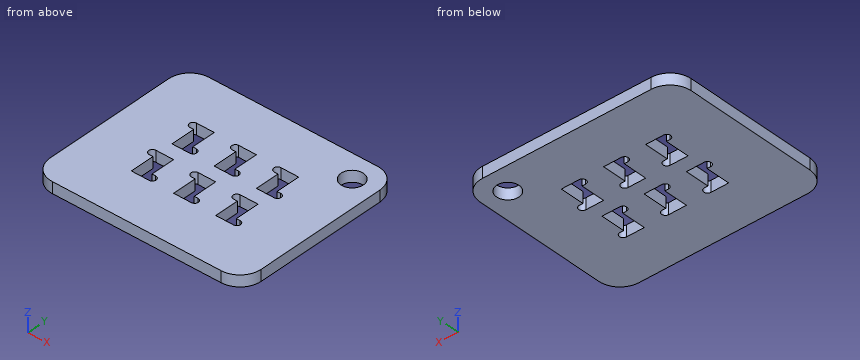
from build123d import *

# Parameters (mm, degrees)
F0_R     = 1.5875
F1_DEPTH = 1.5875


# Not quite as in the source:
# - a length typed as a fraction of an inch, garbled in the dataset ("3 / 203.2 mm" for 3/8 in), is restored


with BuildPart() as f1:
    # F0 (on Top) → F1 (new body)
    with BuildSketch(Plane.XY):
        with BuildLine():
            Line((-6, -12.5), (18, -12.5))
            ThreePointArc((18, -12.5), (20.1213203436, -11.6213203436), (21, -9.5))
            Line((21, -9.5), (21, 9.5))
            ThreePointArc((21, 9.5), (20.1213203436, 11.6213203436), (18, 12.5))
            Line((18, 12.5), (-6, 12.5))
            ThreePointArc((-6, 12.5), (-8.1213203436, 11.6213203436), (-9, 9.5))
            Line((-9, 9.5), (-9, -9.5))
            ThreePointArc((-9, -9.5), (-8.1213203436, -11.6213203436), (-6, -12.5))
        make_face()
        with BuildLine():
            Line((1.525, -5.5), (1, -5.5))
            Line((1, -5.5), (-1, -5.5))
            Line((-1, -5.5), (-1, -2.05))
            Line((-1, -2.05), (-1.525, -2.05))
            ThreePointArc((-1.525, -2.05), (-2.05, -1.525), (-1.525, -1))
            Line((-1.525, -1), (-1, -1))
            Line((-1, -1), (1, -1))
            Line((1, -1), (1, -4.45))
            Line((1, -4.45), (1.525, -4.45))
            ThreePointArc((1.525, -4.45), (2.05, -4.975), (1.525, -5.5))
        make_face(mode=Mode.SUBTRACT)
        with BuildLine():
            Line((7.525, -5.5), (7, -5.5))
            Line((7, -5.5), (5, -5.5))
            Line((5, -5.5), (5, -2.05))
            Line((5, -2.05), (4.475, -2.05))
            ThreePointArc((4.475, -2.05), (3.95, -1.525), (4.475, -1))
            Line((4.475, -1), (5, -1))
            Line((5, -1), (7, -1))
            Line((7, -1), (7, -4.45))
            Line((7, -4.45), (7.525, -4.45))
            ThreePointArc((7.525, -4.45), (8.05, -4.975), (7.525, -5.5))
        make_face(mode=Mode.SUBTRACT)
        with BuildLine():
            Line((13.525, -5.5), (13, -5.5))
            Line((13, -5.5), (11, -5.5))
            Line((11, -5.5), (11, -2.05))
            Line((11, -2.05), (10.475, -2.05))
            ThreePointArc((10.475, -2.05), (9.95, -1.525), (10.475, -1))
            Line((10.475, -1), (11, -1))
            Line((11, -1), (13, -1))
            Line((13, -1), (13, -4.45))
            Line((13, -4.45), (13.525, -4.45))
            ThreePointArc((13.525, -4.45), (14.05, -4.975), (13.525, -5.5))
        make_face(mode=Mode.SUBTRACT)
        with BuildLine():
            Line((-1, 5.5), (1, 5.5))
            Line((1, 5.5), (1, 2.05))
            Line((1, 2.05), (1.525, 2.05))
            ThreePointArc((1.525, 2.05), (2.05, 1.525), (1.525, 1))
            Line((1.525, 1), (1, 1))
            Line((1, 1), (-1, 1))
            Line((-1, 1), (-1, 4.45))
            Line((-1, 4.45), (-1.525, 4.45))
            ThreePointArc((-1.525, 4.45), (-2.05, 4.975), (-1.525, 5.5))
            Line((-1.525, 5.5), (-1, 5.5))
        make_face(mode=Mode.SUBTRACT)
        with BuildLine():
            Line((7.525, 1), (7, 1))
            Line((7, 1), (5, 1))
            Line((5, 1), (5, 4.45))
            Line((5, 4.45), (4.475, 4.45))
            ThreePointArc((4.475, 4.45), (3.95, 4.975), (4.475, 5.5))
            Line((4.475, 5.5), (5, 5.5))
            Line((5, 5.5), (7, 5.5))
            Line((7, 5.5), (7, 2.05))
            Line((7, 2.05), (7.525, 2.05))
            ThreePointArc((7.525, 2.05), (8.05, 1.525), (7.525, 1))
        make_face(mode=Mode.SUBTRACT)
        with BuildLine():
            Line((13.525, 1), (13, 1))
            Line((13, 1), (11, 1))
            Line((11, 1), (11, 4.45))
            Line((11, 4.45), (10.475, 4.45))
            ThreePointArc((10.475, 4.45), (9.95, 4.975), (10.475, 5.5))
            Line((10.475, 5.5), (11, 5.5))
            Line((11, 5.5), (13, 5.5))
            Line((13, 5.5), (13, 2.05))
            Line((13, 2.05), (13.525, 2.05))
            ThreePointArc((13.525, 2.05), (14.05, 1.525), (13.525, 1))
        make_face(mode=Mode.SUBTRACT)
        with Locations((17.5, 9)):
            Circle(F0_R, mode=Mode.SUBTRACT)
    extrude(amount=F1_DEPTH)


solid = f1.part
Read the model definition and answer for the solid it produces. Units are mm, in the model's axes. Give positions to 0.01 mm unless a question says otherwise; leave off trailing zeros. Write each loop counter-clockwise with the first axis right and the second up, starting at its lowest first coordinate (ties: lowest second). Pieces come first, ordered by that corner, then holes. Notation, with made-up numbers: (46, 9.25) - (77, 9.25) arc R22 ccw to (77, 15.25) - close; hole circle Ø1 at (87, -31.5). An arc over 180 degrees is marked (long way). Return JSON: item names as keys, results as strings.
Q1. A cutting plane is placed at C-C, the plane y = 9. Determine the outline of the cut face in (x, z), and give its area (3 significant figures).
Reply:
{"outline": "(-9, 0) - (15.91, 0) - (15.91, 1.59) - (-9, 1.59) - close; (19.09, 0) - (21, 0) - (21, 1.59) - (19.09, 1.59) - close", "area": "42.6 mm²"}
Q2. A cutting plane is placed at A-A, the plane y = 3.25. Determine the outline of the cut face in (x, z).
Reply:
{"outline": "(-9, 0) - (-1, 0) - (-1, 1.59) - (-9, 1.59) - close; (1, 0) - (5, 0) - (5, 1.59) - (1, 1.59) - close; (7, 0) - (11, 0) - (11, 1.59) - (7, 1.59) - close; (13, 0) - (21, 0) - (21, 1.59) - (13, 1.59) - close"}
Q3. A cutting plane is placed at B-B, the plane x = 17.5. Determine the outline of the cut face in (y, z).
Reply:
{"outline": "(-12.5, 0) - (7.41, 0) - (7.41, 1.59) - (-12.5, 1.59) - close; (10.59, 0) - (12.5, 0) - (12.5, 1.59) - (10.59, 1.59) - close"}
Q4. A cutting plane is placed at D-D, the plane z = 0.75. Count the separate pieces of the cut face and the enclosed holes in it, and give its area (3 significant figures).
Reply:
{"separate pieces": "1", "enclosed holes": "7", "area": "669 mm²"}
Q5. Consider line 1 along X through (y, z) = (4.25, 0.75); line 2 along Y through (x, z) = (13.5, 0.8); line 3 along Y through (x, z) = (0, 0.55). Determine where each line is inside the solid, lowest interval first. Write a range as [from, to].
Reply:
{"line 1": "[-9, -1], [1, 5], [7, 11], [13, 21]", "line 2": "[-12.5, -5.5], [-4.45, 1], [2.05, 12.5]", "line 3": "[-12.5, -5.5], [-1, 1], [5.5, 12.5]"}
